from build123d import *

# Parameters (mm, degrees)
SKETCH1_W                                       = 7
SKETCH1_H                                       = 2
BOSS_EXTRUDE1_DEPTH                             = 27.5
CSK_FOR_M3_FLAT_HEAD_MACHINE_SCREW1_D           = 3.4
CSK_FOR_M3_FLAT_HEAD_MACHINE_SCREW1_DEPTH       = 19.9898
CSK_FOR_M3_FLAT_HEAD_MACHINE_SCREW1_CSINK_D     = 6.3
CSK_FOR_M3_FLAT_HEAD_MACHINE_SCREW1_CSINK_ANGLE = 90
CSK_FOR_M3_FLAT_HEAD_MACHINE_SCREW1_TIP         = 1.021463052
SKETCH4_W                                       = 45.5
SKETCH4_H                                       = 6
BOSS_EXTRUDE2_DEPTH                             = 4.5
CSK_FOR_M5_FLAT_HEAD_MACHINE_SCREW1_AT_2_COUNT  = 2
CSK_FOR_M5_FLAT_HEAD_MACHINE_SCREW1_AT_2_PITCH  = 32
CSK_FOR_M5_FLAT_HEAD_MACHINE_SCREW1_AT_3_COUNT  = 2
CSK_FOR_M5_FLAT_HEAD_MACHINE_SCREW1_AT_3_PITCH  = 43.863424399
CSK_FOR_M5_FLAT_HEAD_MACHINE_SCREW1_AT_4_COUNT  = 2
CSK_FOR_M5_FLAT_HEAD_MACHINE_SCREW1_AT_4_PITCH  = 30
CUT_EXTRUDE1_REACH                              = 84.846
CUT_EXTRUDE1_END_RADIUS                         = 30.1625
SKETCH13_R                                      = 5.2
CHAMFER1_SIZE                                   = 1
CHAMFER2_SIZE                                   = 2.517275241


with BuildPart() as part:
    # Sketch1 → Boss-Extrude1 (new, symmetric)
    with BuildSketch(Plane(origin=(0, 0, 0), x_dir=(1, 0, 0), z_dir=(0, 1, 0))):
        with BuildLine():
            Line((-28.75, 16.87680083), (-28.75, 47.337500038))
            Line((-28.75, 47.337500038), (-33.75, 52.337500038))
            Line((-33.75, 52.337500038), (-33.75, 58.337500038))
            Line((-33.75, 58.337500038), (-22.75, 58.337500038))
            Line((-22.75, 58.337500038), (-22.75, 36.3375))
            Line((-22.75, 36.3375), (22.75, 36.3375))
            Line((22.75, 36.3375), (22.75, 42.3375))
            Line((22.75, 42.3375), (33.75, 42.3375))
            Line((33.75, 42.3375), (33.75, 41.680645751))
            Line((33.75, 41.680645751), (25.850505063, 33.781150814))
            Line((25.850505063, 33.781150814), (29.386038969, 30.245616908))
            Line((29.386038969, 30.245616908), (35.75, 36.609577939))
            Line((35.75, 36.609577939), (39.992640687, 32.366937252))
            Line((39.992640687, 32.366937252), (27.075624874, 19.449921438))
            Line((27.075624874, 19.449921438), (26.261945555, 14.835316711))
            ThreePointArc((26.261945555, 14.835316711), (-27.052466926, -13.339431752), (27.757868174, 11.801574499))
            Line((27.757868174, 11.801574499), (28.675140267, 17.00368304))
            Line((28.675140267, 17.00368304), (42.015517583, 30.344060356))
            Line((42.015517583, 30.344060356), (45.551051488, 26.80852645))
            Line((45.551051488, 26.80852645), (31.001655302, 12.259130263))
            ThreePointArc((31.001655302, 12.259130263), (-2.568697776, -33.238391928), (-28.75, 16.87680083))
        make_face()
        with Locations((-28.25, 55.337500038)):
            Rectangle(SKETCH1_W, SKETCH1_H, mode=Mode.SUBTRACT)
    extrude(amount=BOSS_EXTRUDE1_DEPTH, both=True)

    # CSK for M3 Flat Head Machine Screw1
    with Locations(Plane(origin=(9.371262519, 0, 9.371262519), x_dir=(0.7071067811865392, 0, -0.7071067811865558), z_dir=(0.7071067811865558, 0, 0.7071067811865392))):
        with Locations((46.165948244, 20), (46.165948244, 0), (46.165948244, -20)):
            CounterSinkHole(CSK_FOR_M3_FLAT_HEAD_MACHINE_SCREW1_D / 2, CSK_FOR_M3_FLAT_HEAD_MACHINE_SCREW1_CSINK_D / 2, depth=CSK_FOR_M3_FLAT_HEAD_MACHINE_SCREW1_DEPTH, counter_sink_angle=CSK_FOR_M3_FLAT_HEAD_MACHINE_SCREW1_CSINK_ANGLE)
            with Locations((0, 0, -(CSK_FOR_M3_FLAT_HEAD_MACHINE_SCREW1_DEPTH + CSK_FOR_M3_FLAT_HEAD_MACHINE_SCREW1_TIP / 2))):  # 118° drill point
                Cone(0, CSK_FOR_M3_FLAT_HEAD_MACHINE_SCREW1_D / 2, CSK_FOR_M3_FLAT_HEAD_MACHINE_SCREW1_TIP, mode=Mode.SUBTRACT)

    # Sketch4 → Boss-Extrude2 (add)
    with BuildSketch(Plane.XZ.offset(-27.5)):
        with Locations((0, -39.3375)):
            Rectangle(SKETCH4_W, SKETCH4_H)
    extrude(amount=BOSS_EXTRUDE2_DEPTH)

    # Sketch12 → CSK for M5 Flat Head Machine Screw1 (revolve, cut)
    with BuildSketch(Plane(origin=(-16, 15, -30.1625), x_dir=(0, -1, 0), z_dir=(1, 0, 0))):
        Polygon((0, 0), (0, 28.175000038), (2.75, 28.175000038), (2.75, 2.45), (5.2, 0), align=None)
    csk_for_m5_flat_head_machine_screw1 = revolve(axis=Axis((-16, 15, -23.8125), (0, 0, -1)), mode=Mode.SUBTRACT)

    # CSK for M5 Flat Head Machine Screw1 at 2: CSK for M5 Flat Head Machine Screw1 ×2
    with Locations(*[(i * CSK_FOR_M5_FLAT_HEAD_MACHINE_SCREW1_AT_2_PITCH, 0, 0) for i in range(1, CSK_FOR_M5_FLAT_HEAD_MACHINE_SCREW1_AT_2_COUNT)]):
        add(csk_for_m5_flat_head_machine_screw1, mode=Mode.SUBTRACT)

    # CSK for M5 Flat Head Machine Screw1 at 3: CSK for M5 Flat Head Machine Screw1 ×2
    with Locations(*[Vector(0.7295372041400853, -0.6839411288813297, 0) * (i * CSK_FOR_M5_FLAT_HEAD_MACHINE_SCREW1_AT_3_PITCH) for i in range(1, CSK_FOR_M5_FLAT_HEAD_MACHINE_SCREW1_AT_3_COUNT)]):
        add(csk_for_m5_flat_head_machine_screw1, mode=Mode.SUBTRACT)

    # CSK for M5 Flat Head Machine Screw1 at 4: CSK for M5 Flat Head Machine Screw1 ×2
    with Locations(*[(0, -i * CSK_FOR_M5_FLAT_HEAD_MACHINE_SCREW1_AT_4_PITCH, 0) for i in range(1, CSK_FOR_M5_FLAT_HEAD_MACHINE_SCREW1_AT_4_COUNT)]):
        add(csk_for_m5_flat_head_machine_screw1, mode=Mode.SUBTRACT)

    # Cut-Extrude1: up to this cylinder (the profile starts outside it)
    cut_extrude1_end = Plane(origin=(0, 0, 0), z_dir=(0, -1, 0)) * Cylinder(CUT_EXTRUDE1_END_RADIUS, 261.017, mode=Mode.PRIVATE)
    # Sketch13 → Cut-Extrude1 (cut, up to the surface)
    with BuildSketch(Plane.XY.offset(-30.1625), mode=Mode.PRIVATE) as cut_extrude1_sk1:
        with Locations(Location((-16, -15, 0), (0, 0, 180))):
            Circle(SKETCH13_R)
    cut_extrude1_tool1 = extrude(cut_extrude1_sk1.sketch, amount=CUT_EXTRUDE1_REACH, mode=Mode.PRIVATE) - cut_extrude1_end
    add(cut_extrude1_tool1.solids().sort_by_distance((-16, -15, -30.1625))[0], mode=Mode.SUBTRACT)
    # Sketch13 → Cut-Extrude1 (cut, up to the surface)
    with BuildSketch(Plane.XY.offset(-30.1625), mode=Mode.PRIVATE) as cut_extrude1_sk2:
        with Locations(Location((16, -15, 0), (0, 0, 180))):
            Circle(SKETCH13_R)
    cut_extrude1_tool2 = extrude(cut_extrude1_sk2.sketch, amount=CUT_EXTRUDE1_REACH, mode=Mode.PRIVATE) - cut_extrude1_end
    add(cut_extrude1_tool2.solids().sort_by_distance((16, -15, -30.1625))[0], mode=Mode.SUBTRACT)
    # Sketch13 → Cut-Extrude1 (cut, up to the surface)
    with BuildSketch(Plane.XY.offset(-30.1625), mode=Mode.PRIVATE) as cut_extrude1_sk3:
        with Locations(Location((16, 15, 0), (0, 0, 180))):
            Circle(SKETCH13_R)
    cut_extrude1_tool3 = extrude(cut_extrude1_sk3.sketch, amount=CUT_EXTRUDE1_REACH, mode=Mode.PRIVATE) - cut_extrude1_end
    add(cut_extrude1_tool3.solids().sort_by_distance((16, 15, -30.1625))[0], mode=Mode.SUBTRACT)
    # Sketch13 → Cut-Extrude1 (cut, up to the surface)
    with BuildSketch(Plane.XY.offset(-30.1625), mode=Mode.PRIVATE) as cut_extrude1_sk4:
        with Locations(Location((-16, 15, 0), (0, 0, 180))):
            Circle(SKETCH13_R)
    cut_extrude1_tool4 = extrude(cut_extrude1_sk4.sketch, amount=CUT_EXTRUDE1_REACH, mode=Mode.PRIVATE) - cut_extrude1_end
    add(cut_extrude1_tool4.solids().sort_by_distance((-16, 15, -30.1625))[0], mode=Mode.SUBTRACT)

    # Chamfer1
    chamfer1_edges = [part.edges().sort_by_distance(p)[0] for p in [
        (42.015517583, 0, -30.344060356),
        (45.551051488, 0, -26.80852645),
        (25.850505063, 0, -33.781150814),
        (29.386038969, 0, -30.245616908),
        (35.75, 0, -36.609577939),
        (39.992640687, 0, -32.366937252),
    ]]
    chamfer(chamfer1_edges, length=CHAMFER1_SIZE)

    # Chamfer2
    # the kernel refuses this chamfer: 3, 2.517275241 mm, written as the material it adds along each edge
    with BuildSketch(Plane(origin=(31.001655302, -27.5, -12.259130263), x_dir=(0.3214763469276341, 0, 0.9469176090695871), z_dir=(0, 1, 0))) as chamfer2_piece_1:
        with BuildLine():
            Line((3.284174846, 0), (-CHAMFER2_SIZE * 0.442253757678, CHAMFER2_SIZE * 0.896889967468))
            Line((-CHAMFER2_SIZE * 0.442253757678, CHAMFER2_SIZE * 0.896889967468), (0, 0))
            ThreePointArc((0, 0), (1.695572388, 0.040423367), (3.284174846, 0))
        make_face()
    extrude(amount=55)


solid = part.part
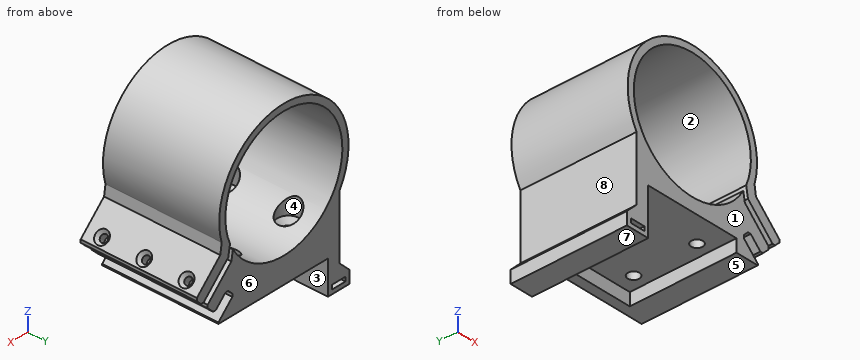
Here's how the part is built. I have some questions about the finished solid (model axes, mm). Face numbers are marked on the shaded views. A direction names the side the tool comes from. Give positions to 0.01 mm unless a question says otherwise; leave off trailing zeros. Loops run counter-clockwise (first coordinate to the right, second up) from the corner with the lowest first, then second, coordinate; pieces in that order, holes last. Notation, with made-up numbers: (80, 67) -> (93, 67) arc R18 ccw to (93, 96) -> close; hole circle Ø1 at (-26.75, 69.5). An arc over 180 degrees is marked (long way). One line per item, written item: value.
Q1. On a 3-axis mill with a long thin cutter (end or side, diameter ignored), from which of +Z, -Z, +X, -X, +Y, -Y can I reach the whole of each face in a straight line? I mean the marked faces 1, 2, 3, 4 and 5. Say none if no direction works.
Answers follow:
face 1: +Z, -Z, +X, -X, -Y
face 2: +Y, -Y
face 3: -Z, -Y
face 4: none
face 5: -Z, +X, +Y, -Y
Q2. Suppose I cut it at A-A on x = 0. Please give me the cut outline in (y, z), then the cut area to 3 significant figures.
Answers follow:
outline: (-27.5, -36.34) -> (23, -36.34) -> (23, -42.34) -> (27.5, -42.34) -> (27.5, -30.16) -> (-27.5, -30.16) -> close; (-27.5, 30.16) -> (27.5, 30.16) -> (27.5, 33.34) -> (-27.5, 33.34) -> close
area: 541 mm^2
Q3. I'm going to push flat-ended pins straight in: pin 1 Ø6.5 at (x, z) = (5.5, -39.5) entering from -Y; pin 2 Ø1.6 at (x, y) = (42, 10) entering from -Z; pin 3 Ø6.5 at (x, y) = (-16, 15) entering from -Z; pin 4 Ø3 at (y, z) = (-5.5, 0.5) entering from -X. Where does each tip first touch, or does it pass through?
Answers follow:
pin 1: y = -27.5
pin 2: z = -29.64
pin 3: z = -36.34
pin 4: x = -33.34
Q4. We'd pull the mould along Z, two halves only. Please class the marked faces 6, 7 and 8: pulls with the +Z half, pulls with the -Z half, needs draft (parallel to the pull), parting line crosses it, or undercut.
Answers follow:
face 6: needs draft
face 7: pulls with the -Z half
face 8: undercut
Q5. Suppose I cut it at D-D on x = 16. Please give me the cut outline in (y, z).
Answers follow:
outline: (-27.5, -36.34) -> (-17.75, -36.34) -> (-17.75, -32.61) -> (-20.2, -30.16) -> (-20.2, -25.57) -> (-27.5, -25.57) -> close; (-27.5, 25.57) -> (27.5, 25.57) -> (27.5, 29.25) -> (-27.5, 29.25) -> close; (-12.25, -36.34) -> (12.25, -36.34) -> (12.25, -32.61) -> (9.8, -30.16) -> (9.8, -25.57) -> (-9.8, -25.57) -> (-9.8, -30.16) -> (-12.25, -32.61) -> close; (17.75, -36.34) -> (23, -36.34) -> (23, -42.34) -> (27.5, -42.34) -> (27.5, -25.57) -> (20.2, -25.57) -> (20.2, -30.16) -> (17.75, -32.61) -> close
Q6. If I drill on line 1 along Y through (x, z) = (-16, -34); line 2 along Y through (x, z) = (16, -26); line 3 along X through (y, z) = (-15, -25.75), over which ranges is the centre line in solid material (lowest first)?
Answers follow:
line 1: -27.5 to -17.75, -12.25 to 12.25, 17.75 to 27.5
line 2: -27.5 to -20.2, -9.8 to 9.8, 20.2 to 27.5
line 3: -28.75 to -21.2, 21.2 to 33.38, 37.42 to 44.49
Q7. Suppose I cut it at B-B on z = 0. Please give me the cut outline in (x, y), then the cut area to 3 significant figures.
Answers follow:
outline: (-33.34, -27.5) -> (-30.16, -27.5) -> (-30.16, 27.5) -> (-33.34, 27.5) -> close; (30.16, -27.5) -> (33.34, -27.5) -> (33.34, 27.5) -> (30.16, 27.5) -> close
area: 349 mm^2
